For this review, use the dimensioned drawing (mm, ordinates from the lowest corner) and the shaded views. Give positions to 0.01 mm unless a question says otherwise; leave off trailing zeros. Loops run counter-clockwise (first coordinate to the right, second up) from the corner with the lowest first, then second, coordinate; pieces in that order, holes last. Notation, with made-up numbers: (-24, 46.5) - (12, 46.5) arc R25 cw to (12, 71.5) - close; hole circle Ø3 at (44, 19). An arc over 180 degrees is marked (long way). Put each result on its own line as item: value.
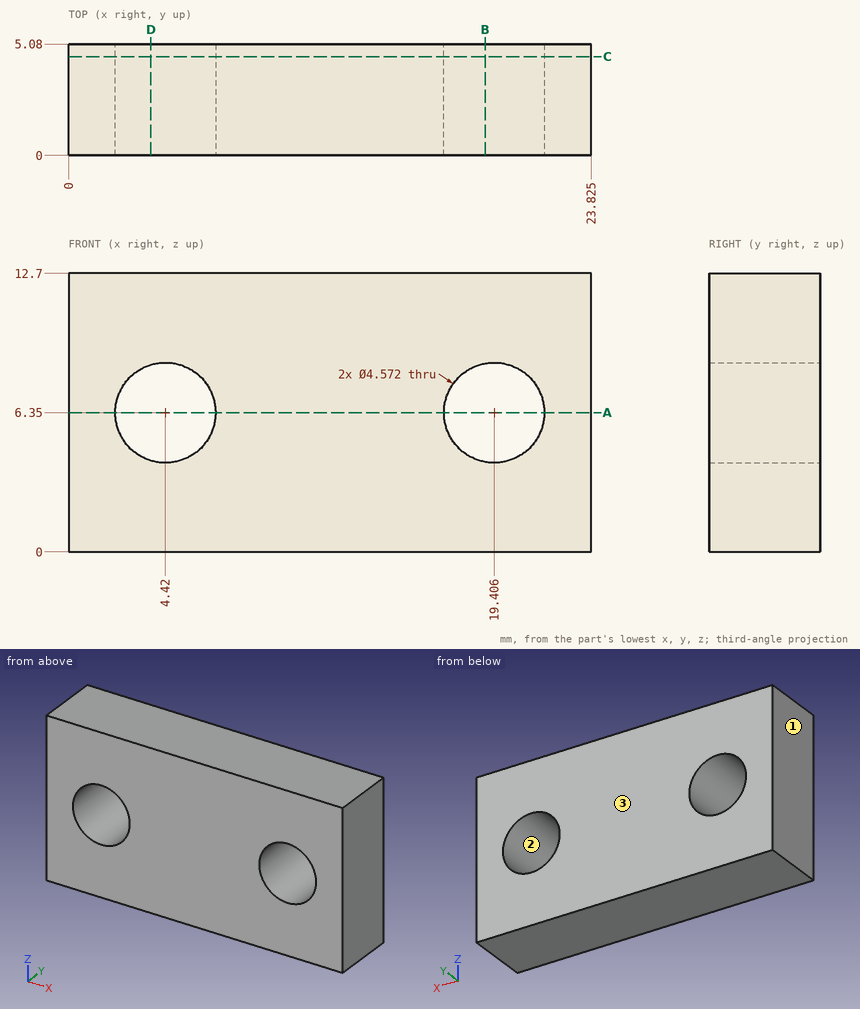
1) Draft analysis for pull direction X (two halves, no side actions). For the marked faces 1, 2 and 3, state which applies: pulls with the +X half, pulls with the -X half, needs draft (parallel to the pull), parting line crosses it, or undercut.
Geometry check:
face 1: pulls with the -X half
face 2: undercut
face 3: needs draft
2) Wall thickness on line 1 (X direction, y = 2.4, z = 6.35) (1 decimal); line 2 (Z direction, x = 4.5, y = 3) (1 decimal); line 3 (X direction, y = 0.5, z = 5.75) (1 decimal): over which ranges is each line inside the solid? List them lowest first.
Geometry check:
line 1: x = 0 to 2.1, 6.7 to 17.1, 21.7 to 23.8
line 2: z = 0 to 4.1, 8.6 to 12.7
line 3: x = 0 to 2.2, 6.6 to 17.2, 21.6 to 23.8
3) Take a section at B-B on x = 19. State the section outline as (y, z) points.
Geometry check:
outline: (0, 0) - (5.08, 0) - (5.08, 4.1) - (0, 4.1) - close; (0, 8.6) - (5.08, 8.6) - (5.08, 12.7) - (0, 12.7) - close
4) Insertion check: pin 1 Ø2.5 at (x, z) = (4.42, 6.35) entering from +Y. The pin has a flat end and moves straight along its axis. Give the tip position at first contact, or say it passes through.
Geometry check:
pin 1: passes through
5) Take a section at D-D on x = 3.75. State the section outline as (y, z) points (1 decimal).
Geometry check:
outline: (0, 0) - (5.1, 0) - (5.1, 4.2) - (0, 4.2) - close; (0, 8.5) - (5.1, 8.5) - (5.1, 12.7) - (0, 12.7) - close
6) Take a section at C-C on y = 4.5. State how many separate pieces and enclosed holes the cut face has, and give its area (3 significant figures).
Geometry check:
separate pieces: 1
enclosed holes: 2
area: 270 mm²
7) Take a section at A-A on z = 6.35. State the section outline as (x, y) points (1 decimal).
Geometry check:
outline: (0, 0) - (2.1, 0) - (2.1, 5.1) - (0, 5.1) - close; (6.7, 0) - (17.1, 0) - (17.1, 5.1) - (6.7, 5.1) - close; (21.7, 0) - (23.8, 0) - (23.8, 5.1) - (21.7, 5.1) - close
